Autodesk Inventor part; units mm, degrees
ref_plane "YZ Plane" through (0, 0, 0) normal (1, 0, 0) x (0, 1, 0)
ref_plane "XZ Plane" through (0, 0, 0) normal (0, 1, 0) x (-1, 0, 0)
ref_plane "XY Plane" through (0, 0, 0) normal (0, 0, 1) x (1, 0, 0)
sketch "Sketch1" plane through (0, 0, 0) normal (1, 0, 0) x (0, 1, 0)
  line L0 (1.6864, 14.4503) -> (11.8425, 14.4503)
  line L1 (11.8425, 14.4503) -> (18.604, 12.6385)
  line L2 (18.604, 12.6385) -> (13.6864, -5.714)
  line L3 (13.6864, -5.714) -> (1.6864, -5.714)
  line L4 (1.6864, -5.714) -> (1.6864, 14.4503)
  point P0 (0, 0)
  dimension "d0" = 19
  dimension "d1" = 7
  dimension "d2" = 105
  dimension "d3" = 12
extrude "Extrusion1" add sketch "Sketch1" along normal blind 19
sketch "Sketch2" plane through (0, 1.6864, -5.714) normal (0, -1, 0) x (1, 0, 0)
  line L0 (0, 0) -> (19, 0)
  line L1 (26.5, -16.4545) -> (10.0455, -25.9545)
  line L2 (0, 0) -> (0, 20.1643) construction
  line L3 (0.5455, -9.5) -> (10.0455, -25.9545)
  line L4 (-2, 0) -> (17, 0)
  line L5 (-2, 0) -> (0.5455, -9.5)
  line L6 (17, 0) -> (26.5, -16.4545)
  line L7 (17, 0) -> (0.5455, -9.5) construction
  point P0 (0, 5.714)
  dimension "d6" = 19
  dimension "d10" = 19
  dimension "d23" = 19
  dimension "d25" = 30
  dimension "d26" = 19
  dimension "d27" = 2
extrude "Extrusion2" add sketch "Sketch2" against normal blind 12
sketch "Sketch3" plane through (26.5, 1.6864, -22.1685) normal (0.8660254, 0, 0.5) x (0.5, 0, -0.8660254)
  line L0 (0, 0) -> (0, 10)
  line L1 (0, 10) -> (0, 15.9167) construction
  line L2 (0, 15.9167) -> (12.6883, 10) construction
  line L3 (12.6883, 10) -> (20.7181, 27.2198)
  line L4 (20.7181, 27.2198) -> (29.7811, 22.9937)
  line L5 (29.7811, 22.9937) -> (29.7811, 0)
  line L6 (29.7811, 0) -> (0, 0)
  line L7 (0, 10) -> (12.6883, 10)
  line L8 (0, 0) -> (0, 12)
  dimension "d16" = 19
  dimension "d17" = 10
  dimension "d18" = 14
  dimension "d20" = 25
  dimension "d30" = 10
extrude "Extrusion4" add sketch "Sketch3" against normal blind 19
shell "Shell1" thickness 2.5 removed faces 1 at (27.7756, 1.6864, -37.0445)
sketch "Sketch4" plane through (0, 18.604, 12.6385) normal (0, 0.9659258, -0.258819) x (1, 0, 0)
  line L0 (2.5, 2.5) -> (16.5, 2.5)
  line L1 (16.5, 17.0817) -> (16.5, 2.5)
  line L2 (2.5, 2.5) -> (16.5, 2.5)
  line L3 (16.5, 2.5) -> (16.5, 17.0817)
  line L4 (16.5, 17.0817) -> (2.5, 17.0817)
  line L5 (2.5, 17.0817) -> (2.5, 2.5)
  point P0 (0, 17.023)
sketch "Sketch5" plane through (0, 13.6864, -5.714) normal (0, 1, 0) x (1, 0, 0)
  line L0 (23.0849, 15.5394) -> (10.9606, 22.5394)
  line L1 (10.9606, 22.5394) -> (23.0849, 15.5394)
  line L2 (23.0849, 15.5394) -> (16.0849, 3.4151)
  line L3 (16.0849, 3.4151) -> (3.9606, 10.4151)
  line L4 (3.9606, 10.4151) -> (10.9606, 22.5394)
  point P0 (0, -5.714)
  dimension "d32" = 14
sketch "Sketch6" plane through (32.8442, 11.6864, -33.1569) normal (-0.4531539, 0.4226183, 0.7848856) x (0.8660254, 0, 0.5)
  line L0 (-16.5, 16.5) -> (-2.5, 16.5)
  line L1 (-2.5, 16.5) -> (-2.5, 2.5)
  line L2 (-2.5, 2.5) -> (-16.5, 2.5)
  line L3 (-16.5, 2.5) -> (-16.5, 16.5)
  line L4 (0, 19) -> (-19, 19)
  line L5 (-19, 0) -> (-19, 19)
  point P0 (-11.8654, -29.6671)
  dimension "d33" = 14
  dimension "d34" = 14
  dimension "d35" = 2.5
  dimension "d36" = 2.5
extrude "Extrusion5" cut sketch "Sketch4" against normal up to next
extrude "Extrusion6" cut sketch "Sketch5" against normal up to next
extrude "Extrusion7" cut sketch "Sketch6" against normal up to next
properties part number "k2_thumb"
CAD build for the part. Positions are in the model's coordinates, mm. A direction names the side the tool comes from. Coordinates: 2 decimals unless noted, no trailing zeros. Order: outer loops, then holes, each group sorted by start corner. A loop starts at its lowest first (then second) coordinate and runs counter-clockwise, first axis right, second up. Notation, with made-up numbers: (18.5, -25.75) -> (33.5, -25.75) arc R16 ccw to (33.5, -8.75) -> close; hole circle Ø4 at (25.25, 24.5). An arc over 180 degrees is marked (long way). Answer in a Markdown table with one row per item.
1) Band-saw the part on B-B (z = -12.5). List the corners of the cut face in (x, y).
Check values:
| item | result |
|---|---|
| outline | (-0.18, 1.69) -> (2.41, 1.69) -> (2.41, 11.19) -> (10.25, 11.19) -> (10.25, 13.69) -> (-0.18, 13.69) -> close; (18.03, 1.69) -> (20.92, 1.69) -> (20.92, 13.69) -> (18.03, 13.69) -> close |
2) Which spindle directions (+Z, -Z, +X, -X, +Y, -Y) get a long thin tool onto all of the face, cutting with end or side? Do faces 5 (the face through (8, 13.686, -13)), 6 (the face through (9.6, 12.99, -3.54)), 7 (the face through (2.055, 6.37, -11.189)). Say none if no direction does.
Check values:
| item | result |
|---|---|
| face 5 | +X, -X, +Y |
| face 6 | +Y |
| face 7 | -Y |
3) Band-saw the part on D-D (z = -52.5). List the corners of the cut face in (x, y), and give its area (3 significant figures).
Check values:
| item | result |
|---|---|
| outline | (22.07, 1.69) -> (24.96, 1.69) -> (24.96, 23.92) -> (28.53, 23.09) -> (28.53, 1.69) -> (33.53, 1.69) -> (33.53, 24.68) -> (22.07, 27.35) -> close |
| area | 201 mm2 |
4) Band-saw the part on C-C (y = 7.5). List the corners of the cut face in (x, z).
Check values:
| item | result |
|---|---|
| outline | (-2, -5.71) -> (0.55, -15.21) -> (10.05, -31.67) -> (24.94, -57.46) -> (41.39, -47.96) -> (26.5, -22.17) -> (17, -5.71) -> (19, -5.71) -> (19, 14.45) -> (0, 14.45) -> (0, -5.71) -> close; hole (1.26, -8.21) -> (2.88, -14.25) -> (12.21, -30.42) -> (25.85, -54.04) -> (37.98, -47.04) -> (24.33, -23.42) -> (12.67, -3.21) -> (16.5, -3.21) -> (16.5, 11.95) -> (2.5, 11.95) -> (2.5, -8.21) -> close |
5) Flat gauge pins, fed straight in: P1, Ø4, axis at x = 16, y = 24, coming from the -Z side; P2, Ø1, axis at x = 2, y = 4, coming from the -Z side; P3, Ø10, axis at x = 18.5, z = -27.5, coming from the +Y side; P4, Ø1, axis at y = 15.5, z = -50, coming from the -X side. Where does each tip first touch, or does it go through?
Check values:
| item | result |
|---|---|
| P1 | through |
| P2 | z = -18.6 |
| P3 | y = 13.69 |
| P4 | x = 20.34 |
6) Drill centre lines: line 1 (X direction, y = 16, z = 5); line 2 (Y direction, x = 25, z = -25.5); line 3 (Z direction, x = 37, y = 22.75). Where is each one in solid material? Low to high.
Check values:
| item | result |
|---|---|
| line 1 | 0 to 2.5, 16.5 to 19 |
| line 2 | 9.19 to 11.69 |
| line 3 | -50.49 to -47.61, -45.36 to -40.36 |
7) Band-saw the part on A-A (x = 9). List the corners of the cut face in (y, z).
Check values:
| item | result |
|---|---|
| outline | (1.69, -29.86) -> (13.69, -29.86) -> (13.69, -24.86) -> (1.69, -24.86) -> close; (1.69, 11.95) -> (11.51, 11.95) -> (15.54, 10.87) -> (17.96, 10.22) -> (18.6, 12.64) -> (11.84, 14.45) -> (1.69, 14.45) -> close; (11.19, -13.22) -> (13.69, -13.22) -> (13.69, -5.71) -> (14.18, -3.86) -> (11.77, -3.21) -> (11.19, -5.38) -> close |
8) Mould opens along Z. For faces 1 (the face through (33.278, 13.344, -52.643)), 2 (the face through (2.5, 8, 2)), 3 (the face through (0, 8, 5)), 4 (the face through (22, 11.686, -32)) say: pulls with the +Z half, pulls with the -Z half, needs draft (parallel to the pull), parting line crosses it, or undercut.
Check values:
| item | result |
|---|---|
| face 1 | pulls with the -Z half |
| face 2 | undercut |
| face 3 | needs draft |
| face 4 | undercut |
